Part model, mm, in its own coordinate system. Face numbers are marked on the shaded views. A direction names the side the tool comes from. Round coordinates to 2 decimals unless told otherwise and drop trailing zeros. Write each loop counter-clockwise with the first axis right and the second up, starting at its lowest first coordinate (ties: lowest second). Pieces come first, ordered by that corner, then holes. Notation, with made-up numbers: M 36,-28 L 88,-28 A20 ccw 88,11 Z; hole C 3,49.25 d8. An arc over 180 degrees is marked long. Use one line per item in the form item = value. Start each with the question number.
Item 1: Cut at D-D, the plane y = 7.75. Give the cut face in (x, z), then the cut area to 3 significant figures.
Item 2: Flat gauge pins, fed straight in: pin 1 Ø3 at (y, z) = (-7, 5.5) entering from -X; pin 2 Ø3 at (x, z) = (-0.5, 5) entering from -Y; pin 3 Ø3 at (y, z) = (-4, 3) entering from +X. Where does each tip first touch, or does it go through?
Item 3: Mould opens along Z. For the marked faces 3, 4 and 5 say: +Z half, -Z half, draft (parallel to the pull), parting line (faces both ways), or undercut.
Item 4: Cut at A-A, the plane y = 0. Give the cut face in (x, z).
Item 5: Cut at C-C, the plane x = 8.25. Give the cut face in (y, z), then the cut area to 3 significant figures.
Item 6: Probe L1, parallel to Z at x = -1, y = -7.5; L2, parallel to Y at x = 0.75, z = 2.25; L3, parallel to Y at x = 5.75, z = 3.75. List the from-to ranges inside material, lowest first.
Item 7: Which spindle directions (+Z, -Z, +X, -X, +Y, -Y) get a long thin tool onto all of the face, cutting with end or side? Do the marked faces 1 and 2. Say none if no direction does.
from build123d import *

# Parameters (mm, degrees)
CYLINDER_R        = 0.6
CYLINDER_DEPTH    = 7.6
ARRAY_COUNT       = 20
CYLINDER001_R     = 6.1
CYLINDER001_DEPTH = 7.6
SKETCH_R          = 9
PAD_DEPTH         = 0.7
SKETCH001_R       = 9
PAD001_DEPTH      = 0.7
SKETCH002_R       = 4.5
POCKET_DEPTH      = 9.001


with BuildPart() as array:
    # Cylinder → Cylinder (new body)
    with BuildSketch(Plane(origin=(6.1, 0, 0), x_dir=(1, 0, 0), z_dir=(0, 0, 1))):
        Circle(CYLINDER_R)
    extrude(amount=CYLINDER_DEPTH)

    # Array: Array ×20 about axis
    array_axis = Axis((0, 0, 0), (0, 0, 1))


with BuildPart() as array_1:
    add(array.part)
    for i in range(1, ARRAY_COUNT):
        add(array.part.rotate(array_axis, i * 360 / ARRAY_COUNT))


with BuildPart() as pocket:
    # Cylinder001 → Cylinder001 (new body)
    with BuildSketch(Plane.XY):
        Circle(CYLINDER001_R)
    extrude(amount=CYLINDER001_DEPTH)

    # Cut: cut Array
    add(array_1.part, mode=Mode.SUBTRACT)


with BuildPart() as pocket_1:
    # Cut placement: moved
    add(pocket.part.moved(Location((0, 0, 1))))

    # Sketch → Pad (new body)
    with BuildSketch(Plane.XY.offset(8.6)):
        Circle(SKETCH_R)
    extrude(amount=PAD_DEPTH)

    # Sketch001 → Pad001 (new body)
    with BuildSketch(Plane(origin=(0, 0, 1), x_dir=(1, 0, 0), z_dir=(0, 0, -1))):
        Circle(SKETCH001_R)
    extrude(amount=PAD001_DEPTH)

    # Sketch002 → Pocket (cut, through all)
    with BuildSketch(Plane.XY.offset(9.3)):
        Circle(SKETCH002_R)
    extrude(amount=-POCKET_DEPTH, mode=Mode.SUBTRACT)


solid = pocket_1.part
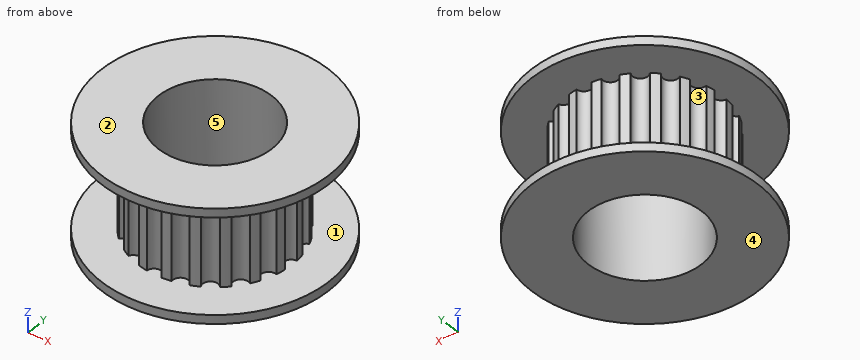
Model answer:
q1.outline = M -4.58,0.3 L 4.58,0.3 L 4.58,1 L -4.58,1 Z; M -4.58,8.6 L 4.58,8.6 L 4.58,9.3 L -4.58,9.3 Z
q1.area = 12.8 mm²
q2.pin_1 = -2.64
q2.pin_2 = -6.07
q2.pin_3 = 5.56
q3.face_3 = undercut
q3.face_4 = -Z half
q3.face_5 = draft
q4.outline = M -9,0.3 L -4.5,0.3 L -4.5,9.3 L -9,9.3 L -9,8.6 L -5.5,8.6 L -5.5,1 L -9,1 Z; M 4.5,0.3 L 9,0.3 L 9,1 L 5.5,1 L 5.5,8.6 L 9,8.6 L 9,9.3 L 4.5,9.3 Z
q5.outline = M -3.6,0.3 L 3.6,0.3 L 3.6,1 L -3.6,1 Z; M -3.6,8.6 L 3.6,8.6 L 3.6,9.3 L -3.6,9.3 Z
q5.area = 10.1 mm²
q6.L1 = 0.3 to 1, 8.6 to 9.3
q6.L2 = -6.05 to -4.44, 4.44 to 6.05
q6.L3 = -1.29 to -0.49, 0.49 to 1.29
q7.face_1 = none
q7.face_2 = +Z, +X, -X, +Y, -Y
